Can you work these out from the model? Positions are in its coordinate system, mm. Round coordinates to 2 decimals unless told otherwise and drop trailing zeros. Loops run counter-clockwise (first coordinate to the right, second up) from the corner with the lowest first, then second, coordinate; pieces in that order, holes last. Notation, with made-up numbers: M 14.25,33.5 L 18.25,33.5 A17 ccw 18.25,58.5 Z; hole C 53.25,-0.75 d3. An arc over 180 degrees is marked long. Return JSON: item names as keys, results as strings.
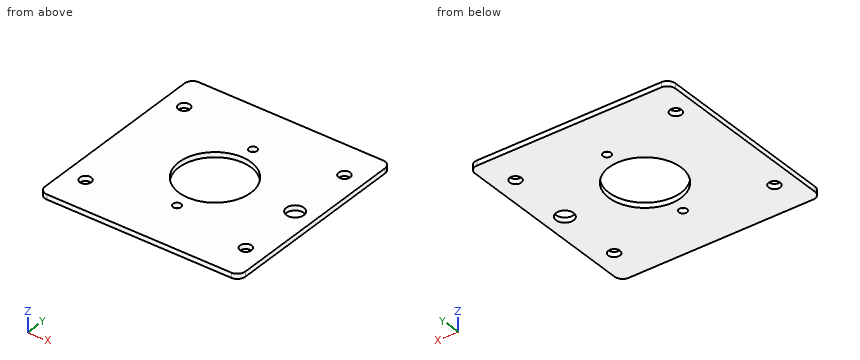
```python
from build123d import *

# Parameters (mm, degrees)
SKETCH3_W                       = 63.5
SKETCH3_H                       = 1.5875
BASE_FLANGE1_DEPTH              = 31.75
FILLET1_R                       = 2.54
F_27_0_144_DIAMETER_HOLE1_D     = 3.6576
SKETCH10_R                      = 11.43
SKETCH10_R_2                    = 1.27
CUT_EXTRUDE1_DEPTH              = 45.929335141
F_7_32_0_21875_DIAMETER_HOLE1_D = 5.55625


# Sheet-metal steps are written as plain solids
with BuildPart() as part:
    # Sketch3 → Base-Flange1 (new, symmetric)
    with BuildSketch(Plane(origin=(0, 0, 0), x_dir=(-1, 0, 0), z_dir=(0, 1, 0))):
        with Locations((0, -0.79375)):
            Rectangle(SKETCH3_W, SKETCH3_H)
    extrude(amount=BASE_FLANGE1_DEPTH, both=True)

    # Fillet1
    fillet1_edges = [part.edges().sort_by_distance(p)[0] for p in [
        (31.75, 31.75, -0.79375),
        (31.75, -31.75, -0.79375),
        (-31.75, -31.75, -0.79375),
        (-31.75, 31.75, -0.79375),
    ]]
    fillet(fillet1_edges, radius=FILLET1_R)

    # #27 (0.144) Diameter Hole1 (through all)
    with Locations(Plane.XY):
        with Locations((-25.4, 20.6375), (25.4, 20.6375), (25.4, -20.6375), (-25.4, -20.6375)):
            Hole(F_27_0_144_DIAMETER_HOLE1_D / 2)

    # Sketch10 → Cut-Extrude1 (cut, through all)
    with BuildSketch(Plane.XY):
        Circle(SKETCH10_R)
        with Locations((0, 15.875)):
            Circle(SKETCH10_R_2)
        with Locations(Location((0, -15.875, 0), (0, 0, 180))):
            Circle(SKETCH10_R_2)
    extrude(amount=-CUT_EXTRUDE1_DEPTH, mode=Mode.SUBTRACT)

    # 7/32 (0.21875) Diameter Hole1 (through all)
    with Locations(Plane.XY):
        with Locations((25.4, 0)):
            Hole(F_7_32_0_21875_DIAMETER_HOLE1_D / 2)


solid = part.part
```
Q1. If I drill on line 1 along Y through (x, z) = (0, -0.95) (3 decimals); line 2 along Y through (x, z) = (25.4, -0.6); line 3 along X through (y, z) = (21, -0.65), over which ranges is the centre line in solid material (lowest first)?
Results:
{"line 1": "y = -31.75 to -17.145, -14.605 to -11.43, 11.43 to 14.605, 17.145 to 31.75", "line 2": "y = -31.75 to -22.47, -18.81 to -2.78, 2.78 to 18.81, 22.47 to 31.75", "line 3": "x = -31.75 to -27.19, -23.61 to 23.61, 27.19 to 31.75"}
Q2. Suppose I cut it at A-A, the plane x = 0. State how many separate pieces and enclosed holes the cut face has, plus the area to 3 significant figures.
Results:
{"separate pieces": "4", "enclosed holes": "0", "area": "56.5 mm2"}
Q3. Suppose I cut it at B-B, the plane y = 5. Please give me the cut outline in (x, z).
Results:
{"outline": "M -31.75,-1.59 L -10.28,-1.59 L -10.28,0 L -31.75,0 Z; M 10.28,-1.59 L 31.75,-1.59 L 31.75,0 L 10.28,0 Z"}
Q4. Suppose I cut it at C-C, the plane x = -25.4. Please give me the cut outline in (y, z).
Results:
{"outline": "M -31.75,-1.59 L -22.47,-1.59 L -22.47,0 L -31.75,0 Z; M -18.81,-1.59 L 18.81,-1.59 L 18.81,0 L -18.81,0 Z; M 22.47,-1.59 L 31.75,-1.59 L 31.75,0 L 22.47,0 Z"}
Q5. I'm going to push a flat-ended pin straight in: pin 1 Ø3 at (x, y) = (0, -15.875) entering from +Z. Where does the tip first touch, or does it pass through?
Results:
{"pin 1": "stops at z = 0"}
